For this review, use the dimensioned drawing (mm, ordinates from the lowest corner) and the shaded views. A direction names the side the tool comes from. Give positions to 0.01 mm unless a question says otherwise; leave off trailing zeros. Loops run counter-clockwise (first coordinate to the right, second up) from the corner with the lowest first, then second, coordinate; pieces in that order, holes last. Notation, with made-up numbers: (-37, -30) -> (-25, -30) arc R24 ccw to (-25, 0) -> close; hole circle Ø10 at (77, 58). An arc over 180 degrees is marked (long way). Write each question's results on one line, items separated by ' | '. Start each with the question number.
Q1. Wall thickness on L1, parallel to Y at x = 48.15, z = 39.5; L2, parallel to X at y = 1.4, z = 20; L3, parallel to Z at x = 59.3, y = 1.1: over which ranges is each line inside the solid? List them lowest first. Write a range as [from, to].
Q2. Machinability: for the marked faces 4, 5 and 6, which of the approach directions +Z, -Z, +X, -X, +Y, -Y give a long, thin tool a straight path to every point of the face, cutting with its end or side? Answer none if there is none.
Q3. We need section B-B (y = 23.5). Write out the cut boundary in (x, z), plus the area to 3 significant figures.
Q4. Mouldability with a two-part tool opening along X and no side actions: class the marked faces 1, 2 and 3 as released by +X, released by -X, zero draft, split by the parting line, or undercut.
Q5. We need section A-A (x = 59.3). Write out the cut boundary in (y, z).
Q6. Insertion check: pin 1 Ø2.5 at (x, z) = (5.7, 20) entering from +Y; pin 2 Ø4 at (x, y) = (16.85, 39.15) entering from -Z; pin 3 Ø6.5 at (x, z) = (59.3, 5) entering from +Y; pin 4 Ø12 at (y, z) = (28, 20.5) entering from -X. Each pin has a flat end and moves straight along its axis. Give the tip position at first contact, or say it passes through.
Q7. We need section C-C (z = 20.5). Write out the cut boundary in (x, y).
Q8. We need section D-D (x = 29). Write out the cut boundary in (y, z).
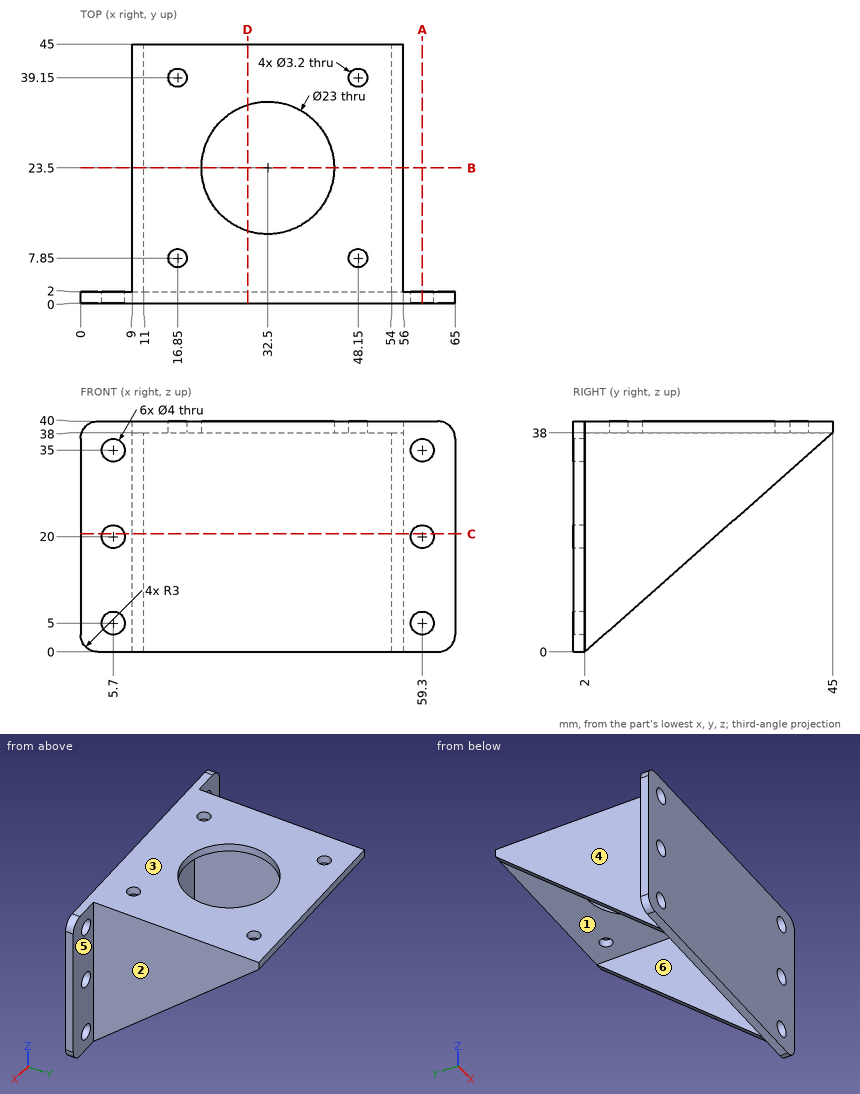
Output:
1) L1: [0, 6.25], [9.45, 37.55], [40.75, 45] | L2: [0, 3.7], [7.7, 57.3], [61.3, 65] | L3: [0, 3], [7, 18], [22, 33], [37, 40]
2) face 4: +Z, -Z, -X, +Y | face 5: +Z, -Z, +X, +Y | face 6: -Z, +Y
3) outline: (9, 19) -> (11, 19) -> (11, 38) -> (21, 38) -> (21, 40) -> (9, 40) -> close; (44, 38) -> (54, 38) -> (54, 19) -> (56, 19) -> (56, 40) -> (44, 40) -> close | area: 124 mm2
4) face 1: undercut | face 2: released by +X | face 3: zero draft
5) outline: (0, 0) -> (2, 0) -> (2, 3) -> (0, 3) -> close; (0, 7) -> (2, 7) -> (2, 18) -> (0, 18) -> close; (0, 22) -> (2, 22) -> (2, 33) -> (0, 33) -> close; (0, 37) -> (2, 37) -> (2, 40) -> (0, 40) -> close
6) pin 1: through | pin 2: z = 38 | pin 3: y = 2 | pin 4: x = 9
7) outline: (0, 0) -> (3.76, 0) -> (3.76, 2) -> (0, 2) -> close; (7.64, 0) -> (57.36, 0) -> (57.36, 2) -> (56, 2) -> (56, 25.2) -> (54, 25.2) -> (54, 2) -> (11, 2) -> (11, 25.2) -> (9, 25.2) -> (9, 2) -> (7.64, 2) -> close; (61.24, 0) -> (65, 0) -> (65, 2) -> (61.24, 2) -> close
8) outline: (0, 0) -> (2, 0) -> (2, 38) -> (12.55, 38) -> (12.55, 40) -> (0, 40) -> close; (34.45, 38) -> (45, 38) -> (45, 40) -> (34.45, 40) -> close
